```python
from build123d import *

# Parameters (mm, degrees)
SKETCH1_R           = 3.5
SKETCH1_R_2         = 1.25
BOSS_EXTRUDE2_DEPTH = 2
BOSS_EXTRUDE3_START = -2
BOSS_EXTRUDE3_DEPTH = 3.5


with BuildPart() as part:
    # Sketch1 → Boss-Extrude2 (new body)
    with BuildSketch(Plane.XY):
        with BuildLine():
            Line((4.197420544, 6.215437295), (4.162047902, 8.420458768))
            Line((4.162047902, 8.420458768), (3.472666725, 8.727391043))
            Line((3.472666725, 8.727391043), (1.81034751, 7.278230684))
            Line((1.81034751, 7.278230684), (1.81034751, 18.65))
            ThreePointArc((1.81034751, 18.65), (0, 20.46034751), (-1.81034751, 18.65))
            Line((-1.81034751, 18.65), (-1.81034751, 4.391485158))
            ThreePointArc((-1.81034751, 4.391485158), (-3.193479033, 3.516275255), (-4.197420544, 2.22354689))
            Line((-4.197420544, 2.22354689), (-4.197420544, -2.22354689))
            ThreePointArc((-4.197420544, -2.22354689), (-3.102034148, -3.597205046), (-1.582253997, -4.478724404))
            Line((-1.582253997, -4.478724404), (-1.582253997, -9.258684619))
            Line((-1.582253997, -9.258684619), (-0.257557826, -7.495576293))
            ThreePointArc((-0.257557826, -7.495576293), (0, -7.5), (0.257557826, -7.495576293))
            Line((0.257557826, -7.495576293), (1.582253997, -9.258684619))
            Line((1.582253997, -9.258684619), (2.32038535, -9.101789957))
            Line((2.32038535, -9.101789957), (2.813434757, -6.952307881))
            ThreePointArc((2.813434757, -6.952307881), (3.050524823, -6.851590932), (3.284016321, -6.74279147))
            Line((3.284016321, -6.74279147), (5.211307253, -7.814668599))
            Line((5.211307253, -7.814668599), (5.821808989, -7.371113124))
            Line((5.821808989, -7.371113124), (5.397958912, -5.206922276))
            ThreePointArc((5.397958912, -5.206922276), (5.573586191, -5.018479548), (5.74263856, -4.824116744))
            Line((5.74263856, -4.824116744), (7.939278142, -5.019425383))
            Line((7.939278142, -5.019425383), (8.316588965, -4.365903867))
            Line((8.316588965, -4.365903867), (7.049126932, -2.561212506))
            ThreePointArc((7.049126932, -2.561212506), (7.132923872, -2.317627458), (7.208306422, -2.071308409))
            Line((7.208306422, -2.071308409), (9.294475714, -1.356277919))
            Line((9.294475714, -1.356277919), (9.373355155, -0.605790169))
            Line((9.373355155, -0.605790169), (7.481436866, 0.527354174))
            ThreePointArc((7.481436866, 0.527354174), (7.458914215, 0.783963475), (7.427592618, 1.039647968))
            Line((7.427592618, 1.039647968), (9.042573998, 2.541382319))
            Line((9.042573998, 2.541382319), (8.809383085, 3.259070153))
            Line((8.809383085, 3.259070153), (6.620138399, 3.524736526))
            ThreePointArc((6.620138399, 3.524736526), (6.495190528, 3.75), (6.362580573, 3.970839767))
            Line((6.362580573, 3.970839767), (7.227129088, 5.999614466))
            Line((7.227129088, 5.999614466), (6.722188648, 6.560407638))
            Line((6.722188648, 6.560407638), (4.614157861, 5.912659912))
            ThreePointArc((4.614157861, 5.912659912), (4.408389392, 6.067627458), (4.197420544, 6.215437295))
        make_face()
        Circle(SKETCH1_R, mode=Mode.SUBTRACT)
        with Locations((0, 18.65)):
            Circle(SKETCH1_R_2, mode=Mode.SUBTRACT)
    extrude(amount=BOSS_EXTRUDE2_DEPTH)

    # Sketch1<4> → Boss-Extrude3 (add)
    with BuildSketch(Plane.XY.offset(BOSS_EXTRUDE3_START)):
        with BuildLine():
            Line((3.454592444, 4.453459903), (-1.81034751, 4.391485158))
            ThreePointArc((-1.81034751, 4.391485158), (-3.193479033, 3.516275255), (-4.197420544, 2.22354689))
            Line((-4.197420544, 2.22354689), (-4.197420544, -2.22354689))
            ThreePointArc((-4.197420544, -2.22354689), (-3.193479033, -3.516275255), (-1.81034751, -4.391485158))
            Line((-1.81034751, -4.391485158), (3.454592444, -4.453459903))
            Line((3.454592444, -4.453459903), (3.339363392, -2.757369614))
            Line((3.339363392, -2.757369614), (0.868808697, -3.390452986))
            ThreePointArc((0.868808697, -3.390452986), (-3.5, 0), (0.868808697, 3.390452986))
            Line((0.868808697, 3.390452986), (0.896736855, 3.383296353))
            Line((0.896736855, 3.383296353), (3.339363392, 2.757369614))
            Line((3.339363392, 2.757369614), (3.454592444, 4.453459903))
        make_face()
    extrude(amount=BOSS_EXTRUDE3_DEPTH)


solid = part.part
```
Input: part model. Units: mm. Frame: model coordinates. A direction names the side the tool comes from. Round coordinates to 2 decimals unless told otherwise and drop trailing zeros. Write each loop counter-clockwise with the first axis right and the second up, starting at its lowest first coordinate (ties: lowest second). Pieces come first, ordered by that corner, then holes. Notation, with made-up numbers: M 35,18 L 79,18 A21 cw 79,39 Z; hole C 71,-3 d10. An arc over 180 degrees is marked long. Write each question's results on one line, items separated by ' | '.
Q1. Line query: line 1 along Y through (x, z) = (0, 1.05); line 2 along Y through (x, z) = (-0.5, 0.5); line 3 along X through (y, z) = (14.5, 1.35). Output: solid intervals per line, ascending.
Results:
line 1: y = -7.5 to -3.5, 3.5 to 17.4, 19.9 to 20.46 | line 2: y = -7.82 to -3.46, 3.46 to 17.5, 19.8 to 20.39 | line 3: x = -1.81 to 1.81
Q2. Section query D-D (y = 10.5). Return loops of the section in (x, z), and give its area (3 significant figures).
Results:
outline: M -1.81,0 L 1.81,0 L 1.81,2 L -1.81,2 Z | area: 7.24 mm^2
Q3. Pin query (flat end, axial travel): P1, Ø1.6, axis at y = 13.5, z = 1, coming from the -X side; P2, Ø1, axis at y = 13, z = 0.5, coming from the +X side; P3, Ø2, axis at x = 1.5, z = 1.5, coming from the +Y side. Return the tip coordinate at first contact, or that it passes through.
Results:
P1: stops at x = -1.81 | P2: stops at x = 1.81 | P3: stops at y = 20.39
Q4. Draft query along X for faces 6 (the face through (0.911, -8.365, 0.986)), 7 (the face through (-0.93, -8.39, 0.99)), 8 (the face through (0.04, 20.46, 0.99)), 9 (the face through (3.396, 3.594, -1.014)). Return one class per face: released by +X, released by -X, zero draft, split by the parting line, or undercut.
Results:
face 6: undercut | face 7: undercut | face 8: split by the parting line | face 9: released by +X
Q5. Section query C-C (z = 0.8). State how many separate pieces and enclosed holes the cut face has, and give its area (3 significant figures).
Results:
separate pieces: 1 | enclosed holes: 2 | area: 157 mm^2
Q6. Access query for faces 1 (the face through (2.563, -8.042, 0.986)), 2 (the face through (3.398, -3.617, -1.014)), 3 (the face through (-1.582, -7, 1)), 4 (the face through (5.68, 6.24, 0.99)), 5 (the face through (7.73, 3.39, 0.99)). Directions: +Z, -Z, +X, -X, +Y, -Y. A direction counts if a zero-diameter tool reaches every point of the face in a straight line with its end or side. Return the directions, or none.
Results:
face 1: +Z, -Z, -Y | face 2: -Z, +X | face 3: +Z, -Z, -X, -Y | face 4: +Z, -Z, +Y | face 5: +Z, -Z, +X
Q7. Section query B-B (z = -1.7). Return loops of the section in (x, y).
Results:
outline: M -4.2,-2.22 A4.75 ccw -1.81,-4.39 L 3.45,-4.45 L 3.34,-2.76 L 0.87,-3.39 A3.5 cw long 0.87,3.39 L 3.34,2.76 L 3.45,4.45 L -1.81,4.39 A4.75 ccw -4.2,2.22 Z
Q8. Section query A-A (y = 0). Return loops of the section in (x, z).
Results:
outline: M -4.2,-2 L -3.5,-2 L -3.5,2 L -4.2,2 Z; M 3.5,0 L 8.36,0 L 8.36,2 L 3.5,2 Z
